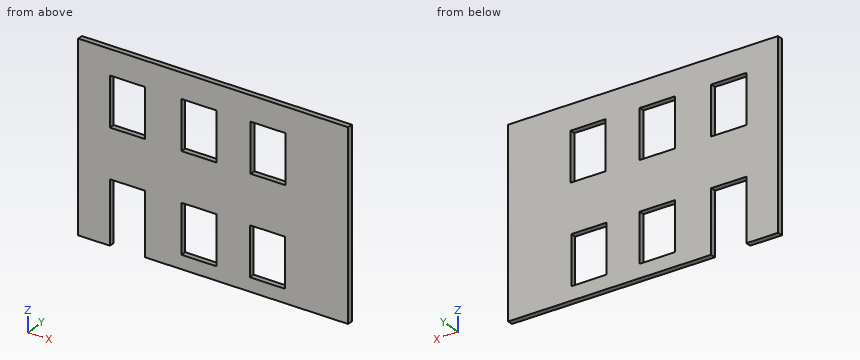
```python
from build123d import *

# Parameters (mm, degrees)
F0_W     = 13
F0_H     = 18
F1_DEPTH = 2


with BuildPart() as f1:
    # F0 (on Front) → F1 (new body)
    with BuildSketch(Plane.XZ):
        Polygon((61.726972, 5.976971), (-38.273028, 5.976971), (-38.273028, -62.023029), (-26.49671, -62.023029), (-26.49671, -39.023029), (-13.49671, -39.023029), (-13.49671, -62.023029), (61.726972, -62.023029), align=None)
        with Locations((6.5, -48.023029)):
            Rectangle(F0_W, F0_H, mode=Mode.SUBTRACT)
        with Locations((31.812498, -48.023029)):
            Rectangle(F0_W, F0_H, mode=Mode.SUBTRACT)
        with Locations((-19.99671, -12.167763)):
            Rectangle(F0_W, F0_H, mode=Mode.SUBTRACT)
        with Locations((6.5, -12.167763)):
            Rectangle(F0_W, F0_H, mode=Mode.SUBTRACT)
        with Locations((32.108551, -12.167763)):
            Rectangle(F0_W, F0_H, mode=Mode.SUBTRACT)
    extrude(amount=F1_DEPTH)


solid = f1.part
```
Source: CAD feature listing. Evaluate the final solid. Frame: model axes, mm. Coordinates: 2 decimals unless noted, no trailing zeros. Loops run counter-clockwise (first coordinate to the right, second up) from the corner with the lowest first, then second, coordinate; pieces in that order, holes last. Notation, with made-up numbers: M 14.25,12.5 L 21.25,12.5 A34 ccw 21.25,50.5 Z; hole C -5,39.25 d6. An arc over 180 degrees is marked long. Put each result on its own line as item: value. Start each with the question number.
1) Cut plane D-D on x = 31. Return the cut outline in (y, z).
2) Cut plane C-C on y = -1.2. Return the cut outline in (x, z).
3) Ray query, L1, parallel to Z at x = 36.5, y = -0.4; L2, parallel to X at y = -0.8, z = -55; L3, parallel to X at y = -0.25, z = -15.5. Return the intervals inside material, ascending. Write a range as from..to.
4) Cut plane B-B on z = -50.5. Return the cut outline in (x, y), then the cut area to 3 significant figures.
5) Cut plane A-A on x = -25.5. Return the cut outline in (y, z), then the cut area to 3 significant figures.
The answers:
1. outline: M -2,-62.02 L 0,-62.02 L 0,-57.02 L -2,-57.02 Z; M -2,-39.02 L 0,-39.02 L 0,-21.17 L -2,-21.17 Z; M -2,-3.17 L 0,-3.17 L 0,5.98 L -2,5.98 Z
2. outline: M -38.27,-62.02 L -26.5,-62.02 L -26.5,-39.02 L -13.5,-39.02 L -13.5,-62.02 L 61.73,-62.02 L 61.73,5.98 L -38.27,5.98 Z; hole M -26.5,-21.17 L -13.5,-21.17 L -13.5,-3.17 L -26.5,-3.17 Z; hole M 0,-57.02 L 13,-57.02 L 13,-39.02 L 0,-39.02 Z; hole M 0,-21.17 L 13,-21.17 L 13,-3.17 L 0,-3.17 Z; hole M 25.31,-57.02 L 38.31,-57.02 L 38.31,-39.02 L 25.31,-39.02 Z; hole M 25.61,-21.17 L 38.61,-21.17 L 38.61,-3.17 L 25.61,-3.17 Z
3. L1: z = -62.02..-57.02, -39.02..-21.17, -3.17..5.98
3. L2: x = -38.27..-26.5, -13.5..0, 13..25.31, 38.31..61.73
3. L3: x = -38.27..-26.5, -13.5..0, 13..25.61, 38.61..61.73
4. outline: M -38.27,-2 L -26.5,-2 L -26.5,0 L -38.27,0 Z; M -13.5,-2 L 0,-2 L 0,0 L -13.5,0 Z; M 13,-2 L 25.31,-2 L 25.31,0 L 13,0 Z; M 38.31,-2 L 61.73,-2 L 61.73,0 L 38.31,0 Z
4. area: 122 mm²
5. outline: M -2,-39.02 L 0,-39.02 L 0,-21.17 L -2,-21.17 Z; M -2,-3.17 L 0,-3.17 L 0,5.98 L -2,5.98 Z
5. area: 54.0 mm²
